Geometry check sheet. Reference: the model listing, model coordinates, mm. Coordinates: 2 decimals unless noted, no trailing zeros. Loops run counter-clockwise (first coordinate to the right, second up) from the corner with the lowest first, then second, coordinate; pieces in that order, holes last. Notation, with made-up numbers: (-35.75, 39.5) -> (4.25, 39.5) arc R15 cw to (4.25, 62.5) -> close; hole circle Ø11 at (15.25, 24.25). An arc over 180 degrees is marked (long way). Answer as a JSON object with one key per item and string values.
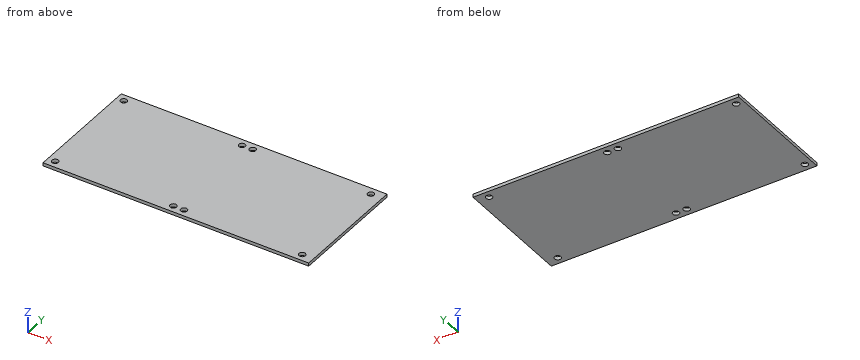
Autodesk Fusion 360 part; units mm, degrees
sketch "Sketch1" plane through (0, 0, 0) normal (0, 0, 1) x (1, 0, 0)
  line L0 (0, 0) -> (50, 0)
  line L1 (50, 0) -> (50, 45)
  line L2 (50, 45) -> (0, 45)
  line L3 (0, 45) -> (0, 0)
  line L4 (47.25, 42.25) -> (2.75, 42.25)
  line L5 (2.75, 42.25) -> (2.75, 2.75)
  line L6 (2.75, 2.75) -> (47.25, 2.75)
  line L7 (47.25, 2.75) -> (47.25, 42.25)
  line L8 (47.25, 42.25) -> (2.75, 2.75) construction
  line L9 (2.75, 42.25) -> (47.25, 2.75) construction
  line L10 (50, 45) -> (0, 0) construction
  circle A0 centre (2.75, 42.25) radius 1.2
  circle A1 centre (2.75, 2.75) radius 1.2
  circle A2 centre (47.25, 42.25) radius 1.2
  circle A3 centre (47.25, 2.75) radius 1.2
  line L11 (95.75, 2.75) -> (95.75, 42.25)
  line L12 (51.25, 2.75) -> (95.75, 2.75)
  line L13 (98.5, 45) -> (48.5, 0) construction
  line L14 (51.25, 42.25) -> (95.75, 2.75) construction
  line L15 (95.75, 42.25) -> (51.25, 2.75) construction
  circle A4 centre (51.25, 42.25) radius 1.2
  circle A5 centre (51.25, 2.75) radius 1.2
  line L16 (95.75, 42.25) -> (51.25, 42.25)
  circle A6 centre (95.75, 42.25) radius 1.2
  circle A7 centre (95.75, 2.75) radius 1.2
  line L17 (51.25, 42.25) -> (51.25, 2.75)
  line L18 (50, 45) -> (100, 45)
  line L19 (100, 45) -> (100, 0)
  line L20 (100, 0) -> (50, 0)
  line L21 (50, 0) -> (50, 45)
  point P0 (25, 22.5)
  point P1 (73.5, 22.5)
  dimension "d1" = 50
  dimension "d2" = 44.5
  dimension "d3" = 39.5
  dimension "d4" = 2.4
  dimension "d5" = 2.4
  dimension "d6" = 2.4
  dimension "d7" = 2.4
  dimension "d12" = 45
  dimension "d14" = 44.5
  dimension "d15" = 39.5
  dimension "d16" = 2.4
  dimension "d17" = 2.4
  dimension "d18" = 2.4
  dimension "d19" = 2.4
  dimension "d22" = 4
  dimension "d23" = 100
  dimension "d24" = 45
  dimension "d25" = 4.25
extrude "Extrude1" add sketch "Sketch1" along normal blind 1.2 contours L0 L1 L2 L3 L21 | L4 L5 L6 L7 A0 A1 A2 A3
extrude "Extrude3" add sketch "Sketch1" along normal blind 1.2 contours L1 L18 L19 L20 L21 | L11 L12 A4 A5 L16 A6 A7 L17
1. Section check B-B, the plane y = 2.75. Record the boundary of the cut face in (x, z).
Evaluation:
{"outline": "(0, 0) -> (1.55, 0) -> (1.55, 1.2) -> (0, 1.2) -> close; (3.95, 0) -> (46.05, 0) -> (46.05, 1.2) -> (3.95, 1.2) -> close; (48.45, 0) -> (50.05, 0) -> (50.05, 1.2) -> (48.45, 1.2) -> close; (52.45, 0) -> (94.55, 0) -> (94.55, 1.2) -> (52.45, 1.2) -> close; (96.95, 0) -> (100, 0) -> (100, 1.2) -> (96.95, 1.2) -> close"}
2. Section check A-A, the plane x = 95.75. Record the boundary of the cut face in (y, z).
Evaluation:
{"outline": "(0, 0) -> (1.55, 0) -> (1.55, 1.2) -> (0, 1.2) -> close; (3.95, 0) -> (41.05, 0) -> (41.05, 1.2) -> (3.95, 1.2) -> close; (43.45, 0) -> (45, 0) -> (45, 1.2) -> (43.45, 1.2) -> close"}
3. Thickness scan on probe 1 along X at (y, z) = (2.75, 0.75); probe 2 along Y at (x, z) = (51.25, 0.9); probe 3 along Y at (x, z) = (48, 1). Record the ranges inside material, lowest first. Write a range as from..to.
Evaluation:
{"probe 1": "x = 0..1.55, 3.95..46.05, 48.45..50.05, 52.45..94.55, 96.95..100", "probe 2": "y = 0..1.55, 3.95..41.05, 43.45..45", "probe 3": "y = 0..1.81, 3.69..41.31, 43.19..45"}
4. Section check C-C, the plane x = 51.5. Record the boundary of the cut face in (y, z).
Evaluation:
{"outline": "(0, 0) -> (1.58, 0) -> (1.58, 1.2) -> (0, 1.2) -> close; (3.92, 0) -> (41.08, 0) -> (41.08, 1.2) -> (3.92, 1.2) -> close; (43.42, 0) -> (45, 0) -> (45, 1.2) -> (43.42, 1.2) -> close"}
5. Depth check by flat-ended pin: P1, Ø1.4, axis at x = 51.25, y = 42.25, coming from the +Z side. Enter the tip coordinate at first touch or a pass-through.
Evaluation:
{"P1": "passes through"}
